Could you check a few things on this model? Use its own coordinates, in mm. Give positions to 0.01 mm unless a question says otherwise; leave off trailing zeros. Write each loop counter-clockwise with the first axis right and the second up, starting at its lowest first coordinate (ties: lowest second). Pieces come first, ordered by that corner, then holes. Notation, with made-up numbers: M 11.5,2 L 31.5,2 A32 ccw 31.5,28 Z; hole C 30.25,66.5 d4. An arc over 180 degrees is marked long. One line per item, written item: value.
```python
from build123d import *

# Parameters (mm, degrees)
SKETCH_1_W          = 117.2
SKETCH_1_H          = 53.16059175
EXTRUDE_1_DEPTH     = 4
SKETCH_3_R          = 1.6
CUT_EXTRUDE_1_DEPTH = 4
FILLET_1_R          = 3
SKETCH_4_R          = 1.6
CUT_EXTRUDE_2_DEPTH = 10


with BuildPart() as part:
    # 草图1 → 凸台-拉伸1 (new body)
    with BuildSketch(Plane(origin=(0, 0, 0), x_dir=(1, 0, 0), z_dir=(0, 1, 0))):
        Rectangle(SKETCH_1_W, SKETCH_1_H)
    extrude(amount=EXTRUDE_1_DEPTH)

    # 草图3 → 切除-拉伸1 (cut)
    with BuildSketch(Plane(origin=(0, 4, 0), x_dir=(1, 0, 0), z_dir=(0, 1, 0))):
        with Locations(Location((-53.6, -21.580295875, 0), (0, 0, 270))):
            Circle(SKETCH_3_R)
        with Locations(Location((-53.6, -13.580295875, 0), (0, 0, 270))):
            Circle(SKETCH_3_R)
        with Locations(Location((-5, -21.580295875, 0), (0, 0, 270))):
            Circle(SKETCH_3_R)
        with Locations(Location((5, -21.580295875, 0), (0, 0, 90))):
            Circle(SKETCH_3_R)
        with Locations(Location((53.6, -13.580295875, 0), (0, 0, 90))):
            Circle(SKETCH_3_R)
        with Locations(Location((53.6, -21.580295875, 0), (0, 0, 90))):
            Circle(SKETCH_3_R)
        with Locations(Location((-53.6, 13.580295875, 0), (0, 0, 90))):
            Circle(SKETCH_3_R)
        with Locations(Location((-53.6, 21.580295875, 0), (0, 0, 90))):
            Circle(SKETCH_3_R)
        with Locations(Location((-5, 21.580295875, 0), (0, 0, 90))):
            Circle(SKETCH_3_R)
        with Locations(Location((5, 21.580295875, 0), (0, 0, 270))):
            Circle(SKETCH_3_R)
        with Locations(Location((53.6, 21.580295875, 0), (0, 0, 270))):
            Circle(SKETCH_3_R)
        with Locations(Location((53.6, 13.580295875, 0), (0, 0, 270))):
            Circle(SKETCH_3_R)
    extrude(amount=-CUT_EXTRUDE_1_DEPTH, mode=Mode.SUBTRACT)

    # 圆角1
    fillet_1_edges = [part.edges().sort_by_distance(p)[0] for p in [
        (58.6, 2, 26.580295875),
        (-58.6, 2, 26.580295875),
        (-58.6, 2, -26.580295875),
        (58.6, 2, -26.580295875),
    ]]
    fillet(fillet_1_edges, radius=FILLET_1_R)

    # 草图4 → 切除-拉伸2 (cut)
    with BuildSketch(Plane(origin=(0, 4, 0), x_dir=(1, 0, 0), z_dir=(0, 1, 0))):
        with Locations(Location((-15, -15, 0), (0, 0, 270))):
            Circle(SKETCH_4_R)
        with Locations(Location((15, 15, 0), (0, 0, 270))):
            Circle(SKETCH_4_R)
        with Locations(Location((15, -15, 0), (0, 0, 270))):
            Circle(SKETCH_4_R)
        with Locations(Location((-15, 15, 0), (0, 0, 270))):
            Circle(SKETCH_4_R)
    extrude(amount=-CUT_EXTRUDE_2_DEPTH, mode=Mode.SUBTRACT)


solid = part.part
```
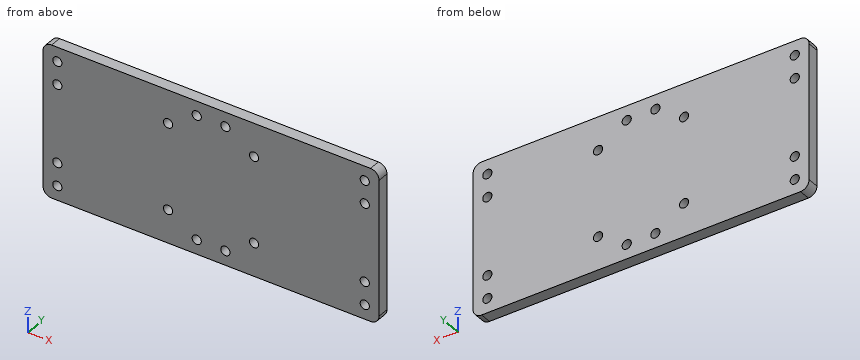
1) If we section it at C-C, the plane x = -53.6: Write out the boundary of the cut face in (y, z).
Outcome:
outline: M 0,-26.58 L 4,-26.58 L 4,-23.18 L 0,-23.18 Z; M 0,-19.98 L 4,-19.98 L 4,-15.18 L 0,-15.18 Z; M 0,-11.98 L 4,-11.98 L 4,11.98 L 0,11.98 Z; M 0,15.18 L 4,15.18 L 4,19.98 L 0,19.98 Z; M 0,23.18 L 4,23.18 L 4,26.58 L 0,26.58 Z
2) Please list where these lines run through material, in increasing order: L1, parallel to X at y = 1, z = -21.5; L2, parallel to X at y = 0.6, z = 22; L3, parallel to X at y = 1.8, z = -13. Write a range as from..to.
Outcome:
L1: x = -58.6..-55.2, -52..-6.6, -3.4..3.4, 6.6..52, 55.2..58.6
L2: x = -58.6..-55.14, -52.06..-6.54, -3.46..3.46, 6.54..52.06, 55.14..58.6
L3: x = -58.6..-55.09, -52.11..52.11, 55.09..58.6
3) I'm going to push a flat-ended pin straight in: pin 1 (5 mm diameter, centred on x = -5, z = 21.58, fed in from +Y). Where does the tip first touch, or does it pass through?
Outcome:
pin 1: stops at y = 4
4) If we section it at A-A, the plane x = 15: Write out the boundary of the cut face in (y, z).
Outcome:
outline: M 0,-26.58 L 4,-26.58 L 4,-16.6 L 0,-16.6 Z; M 0,-13.4 L 4,-13.4 L 4,13.4 L 0,13.4 Z; M 0,16.6 L 4,16.6 L 4,26.58 L 0,26.58 Z
5) If we section it at B-B, the plane y = 1: Give the number of separate pieces and of enclosed holes in the cut face, then the cut area to 3 significant figures.
Outcome:
separate pieces: 1
enclosed holes: 16
area: 6,090 mm^2
